Build history of the part. All positions in model axes, mm. Face numbers are marked on the shaded views. Coordinates: 2 decimals unless noted, no trailing zeros. Order: outer loops, then holes, each group sorted by start corner. A loop starts at its lowest first (then second) coordinate and runs counter-clockwise, first axis right, second up. Notation, with made-up numbers: (55, -6.5) -> (64, -6.5) arc R13 cw to (64, 3.5) -> close; hole circle Ø9 at (40.5, 13). An arc over 180 degrees is marked (long way). Write each question's results on one line, items separated by ' | '.
Autodesk Inventor part; units mm, degrees
ref_plane "YZ Plane" through (0, 0, 0) normal (1, 0, 0) x (0, 1, 0)
ref_plane "XZ Plane" through (0, 0, 0) normal (0, 1, 0) x (-1, 0, 0)
ref_plane "XY Plane" through (0, 0, 0) normal (0, 0, 1) x (1, 0, 0)
sketch "スケッチ1" plane through (0, 0, 0) normal (0, 1, 0) x (-1, 0, 0)
  arc A0 (26.9342, 2.5) -> (27.05, 0) centre (0, 0) ccw
  arc A1 (24.9249, 2.5) -> (25.05, 0) centre (0, 0) ccw
  line L0 (26.9342, 2.5) -> (24.9249, 2.5)
  line L1 (39.5466, 0) -> (-39.5755, 0)
  dimension "d0" = 25.05
  dimension "d1" = 2
  dimension "d2" = 2.5
extrude "押し出し1" add sketch "スケッチ1" along normal blind 20 contours L0 A1 L1 A0 | L1 A1 A0
fillet "フィレット1" radius 2 2 edges at (-25.05, 10, 0) (-24.9249, 10, 2.5)
properties part number "Senban_zigu2"
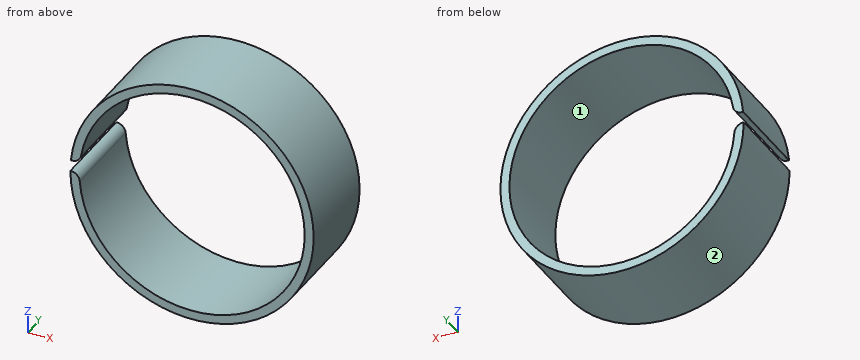
Item 1: Pull direction Z, two halves, no side cores. Call the marked faces 1 and 2: released by +Z, released by -Z, zero draft, split by the parting line, or undercut.
Answer:
face 1: undercut | face 2: split by the parting line
Item 2: Slice it at B-B, the plane x = 7.5. List the corners of the cut face in (y, z).
Answer:
outline: (0, -25.99) -> (20, -25.99) -> (20, -23.9) -> (0, -23.9) -> close; (0, 23.9) -> (20, 23.9) -> (20, 25.99) -> (0, 25.99) -> close
Item 3: Slice it at A-A, the plane z = 22. List the corners of the cut face in (x, y), and give its area (3 significant figures).
Answer:
outline: (-15.74, 0) -> (-11.98, 0) -> (-11.98, 20) -> (-15.74, 20) -> close; (11.98, 0) -> (15.74, 0) -> (15.74, 20) -> (11.98, 20) -> close | area: 150 mm^2
Item 4: Pin check, flat tips, straight feed: pin 1 (8 mm diameter, centred on x = -21, y = 12, fed in from -Z); pin 2 (10 mm diameter, centred on x = 16, y = 9, fed in from +Z); pin 3 (5 mm diameter, centred on x = -18.5, y = 10, fed in from -Z). Stop position of each tip, or through.
Answer:
pin 1: stops at z = -21.04 | pin 2: stops at z = 24.71 | pin 3: stops at z = -21.81
Item 5: Slice it at C-C, the plane y = 10.5. List the corners of the cut face in (x, z), and give its area (3 significant figures).
Answer:
outline: (-27.05, 0) arc R27.05 ccw (long way) to (-26.93, 2.5) -> (-26.67, 2.5) arc R2 ccw to (-24.7, 4.17) arc R25.05 cw (long way) to (-24.98, -1.85) arc R2 ccw to (-26.98, 0) -> close | area: 321 mm^2
Item 6: Drill centre lines: line 1 (Z direction, x = -6.5, y = 1.25); line 2 (Z direction, x = 10.5, y = 2.5); line 3 (X direction, y = 12.5, z = 11). Where is each one in solid material? Low to high. Write a range as from..to.
Answer:
line 1: z = -26.26..-24.19, 24.19..26.26 | line 2: z = -24.93..-22.74, 22.74..24.93 | line 3: x = -24.71..-22.51, 22.51..24.71
